Model file for the job. Use its own axes, mm. A direction names the side the tool comes from. Give positions to 0.01 mm unless a question says otherwise; leave off trailing zeros. Answer as CSV lines item,"result". Start each with the question number.
Item 1: Pull direction X, two halves, no side cores. Call faces 1 (the flat face through (86.43, -55.25, 4.78)), 2 (the flat face through (7.29, 113.98, 1.57)), 3 (the flat face through (-28.156, -69.447, 1.565)): pulls with the +X half, pulls with the -X half, needs draft (parallel to the pull), parting line crosses it, or undercut.
Item 2: Drill centre lines: L1, parallel to Y at x = 56, z = 4.5; L2, parallel to X at y = -35, z = 4; L3, parallel to X at y = 25, z = 5.5 (3 decimals). Where is each one in solid material? Low to high. Write a range as from..to.
Item 3: Tool access for faces 4 (the flat face through (-28.156, -69.447, 4.785)), 5 (the flat face through (86.43, -55.25, 1.57)), 6 (the flat face through (65.881, -68.712, 1.565)), 7 (the flat face through (-77.063, 35.143, 1.565)): list every direction of +Z, -Z, +X, -X, +Y, -Y with a clear straight run to the whole face (end or side of a thin tool).
Item 4: Pin check, flat tips, straight feed: pin 1 (1.5 mm diameter, centred on y = 87, z = 1.5, fed in from +X); pin 2 (2 mm diameter, centred on x = -66, y = 58.5, fed in from -Z); pin 3 (3 mm diameter, centred on x = 50.5, z = 3, fed in from +Y). Stop position of each tip, or through.
from build123d import *

# Parameters (mm, degrees)
F1_DEPTH = 6.35
F2_SIZE  = 3.17499


# Not quite as in the source:
# - a fillet or chamfer is up to 0.001 mm smaller than in the source, because OpenCascade refuses the exact size
# - a feature names something its author has since deleted; it is built from what else it names


with BuildPart() as f1:
    # F0 (on Top) → F1 (new body)
    with BuildSketch(Plane.XY):
        with BuildLine():
            Line((19.3683549781, 156.3463236885), (-8.1032558219, 71.7973993899))
            Line((-8.1032558219, 71.7973993899), (8.3683549781, 71.7973993899))
            ThreePointArc((8.3683549781, 71.7973993899), (11.590180385, 79.5755739829), (19.3683549781, 82.7973993899))
            Line((19.3683549781, 82.7973993899), (19.3683549781, 156.3463236885))
        make_face()
        with BuildLine():
            Line((19.3683549781, 60.7973993899), (19.3683549781, 59.7189816329))
            Line((19.3683549781, 59.7189816329), (38.0644816066, 59.7189816329))
            ThreePointArc((38.0644816066, 59.7189816329), (40.489965778, 67.183854337), (46.839965778, 71.7973993899))
            Line((46.839965778, 71.7973993899), (30.3683549781, 71.7973993899))
            ThreePointArc((30.3683549781, 71.7973993899), (27.1465295711, 64.0192247968), (19.3683549781, 60.7973993899))
        make_face()
        with BuildLine():
            Line((19.3683549781, 59.7189816329), (0.6722283496, 59.7189816329))
            ThreePointArc((0.6722283496, 59.7189816329), (-0.7119887932, 53.9533022862), (-4.5628989463, 49.4444658044))
            Line((-4.5628989463, 49.4444658044), (12.9027172029, 25.4051075068))
            ThreePointArc((12.9027172029, 25.4051075068), (15.96916804, 26.9675422479), (19.3683549781, 27.5059205686))
            Line((19.3683549781, 27.5059205686), (19.3683549781, 59.7189816329))
        make_face()
        with BuildLine():
            ThreePointArc((-4.5628989463, 49.4444658044), (-17.7934509971, 48.4031987757), (-24.7277716504, 59.7189816329))
            Line((-24.7277716504, 59.7189816329), (-29.8177793123, 44.0535488478))
            ThreePointArc((-29.8177793123, 44.0535488478), (-24.3177793123, 40.0575649437), (-22.2169662504, 33.5919271685))
            ThreePointArc((-22.2169662504, 33.5919271685), (-22.3523945039, 31.8711480531), (-22.7553445712, 30.1927402304))
            Line((-22.7553445712, 30.1927402304), (8.9067332988, 19.9051075068))
            ThreePointArc((8.9067332988, 19.9051075068), (10.46916804, 22.9715583438), (12.9027172029, 25.4051075068))
            Line((12.9027172029, 25.4051075068), (-4.5628989463, 49.4444658044))
        make_face()
        with BuildLine():
            Line((-36.6161531886, 23.1303054893), (-41.7061608505, 7.4648727041))
            ThreePointArc((-41.7061608505, 7.4648727041), (-29.4449273159, 12.5436419256), (-19.353227265, 3.9245158286))
            Line((-19.353227265, 3.9245158286), (8.9067332988, 13.1067336305))
            ThreePointArc((8.9067332988, 13.1067336305), (8.3683549781, 16.5059205686), (8.9067332988, 19.9051075068))
            Line((8.9067332988, 19.9051075068), (-22.7553445712, 30.1927402304))
            ThreePointArc((-22.7553445712, 30.1927402304), (-28.2230707533, 23.7908554024), (-36.6161531886, 23.1303054893))
        make_face()
        with BuildLine():
            ThreePointArc((-18.7316450219, 0), (-23.9667723178, -10.2745158286), (-35.3561608505, -12.0784177569))
            Line((-35.3561608505, -12.0784177569), (-22.0303477886, -21.7601876667))
            ThreePointArc((-22.0303477886, -21.7601876667), (-14.8519399659, -17.3612536953), (-6.6655230753, -19.3266385037))
            Line((-6.6655230753, -19.3266385037), (12.9027172029, 7.6067336305))
            ThreePointArc((12.9027172029, 7.6067336305), (10.46916804, 10.0402827934), (8.9067332988, 13.1067336305))
            Line((8.9067332988, 13.1067336305), (-19.353227265, 3.9245158286))
            ThreePointArc((-19.353227265, 3.9245158286), (-18.8880030964, 1.986717706), (-18.7316450219, 0))
        make_face()
        with BuildLine():
            ThreePointArc((19.3683549781, 5.5059205686), (15.96916804, 6.0442988894), (12.9027172029, 7.6067336305))
            Line((12.9027172029, 7.6067336305), (-6.6655230753, -19.3266385037))
            ThreePointArc((-6.6655230753, -19.3266385037), (-3.3300890844, -23.2319299447), (-2.1311608505, -28.2258254419))
            ThreePointArc((-2.1311608505, -28.2258254419), (-2.6695391712, -31.62501238), (-4.2319739124, -34.6914632171))
            Line((-4.2319739124, -34.6914632171), (9.0938391495, -44.3732331268))
            ThreePointArc((9.0938391495, -44.3732331268), (8.0525721209, -31.142681076), (19.3683549781, -24.2083604227))
            Line((19.3683549781, -24.2083604227), (19.3683549781, 5.5059205686))
        make_face()
        with BuildLine():
            Line((45.4022330314, -19.3266385037), (25.8339927533, 7.6067336305))
            ThreePointArc((25.8339927533, 7.6067336305), (22.7675419162, 6.0442988894), (19.3683549781, 5.5059205686))
            Line((19.3683549781, 5.5059205686), (19.3683549781, -24.2083604227))
            ThreePointArc((19.3683549781, -24.2083604227), (28.3486110991, -27.9281043016), (32.0683549781, -36.9083604227))
            ThreePointArc((32.0683549781, -36.9083604227), (31.446772735, -40.8328762512), (29.6428708066, -44.3732331268))
            Line((29.6428708066, -44.3732331268), (42.9686838685, -34.6914632171))
            ThreePointArc((42.9686838685, -34.6914632171), (41.0032990601, -26.5050463264), (45.4022330314, -19.3266385037))
        make_face()
        with BuildLine():
            ThreePointArc((29.8299766573, 13.1067336305), (28.2675419162, 10.0402827934), (25.8339927533, 7.6067336305))
            Line((25.8339927533, 7.6067336305), (45.4022330314, -19.3266385037))
            ThreePointArc((45.4022330314, -19.3266385037), (53.5886499221, -17.3612536953), (60.7670577448, -21.7601876667))
            Line((60.7670577448, -21.7601876667), (74.0928708066, -12.0784177569))
            ThreePointArc((74.0928708066, -12.0784177569), (61.188098857, -8.9802561211), (58.0899372211, 3.9245158286))
            Line((58.0899372211, 3.9245158286), (29.8299766573, 13.1067336305))
        make_face()
        with BuildLine():
            Line((61.4920545274, 30.1927402304), (29.8299766573, 19.9051075068))
            ThreePointArc((29.8299766573, 19.9051075068), (30.2329267246, 18.2266996841), (30.3683549781, 16.5059205686))
            ThreePointArc((30.3683549781, 16.5059205686), (30.2329267246, 14.7851414532), (29.8299766573, 13.1067336305))
            Line((29.8299766573, 13.1067336305), (58.0899372211, 3.9245158286))
            ThreePointArc((58.0899372211, 3.9245158286), (68.1816372721, 12.5436419256), (80.4428708066, 7.4648727041))
            Line((80.4428708066, 7.4648727041), (75.3528631447, 23.1303054893))
            ThreePointArc((75.3528631447, 23.1303054893), (66.9597807095, 23.7908554024), (61.4920545274, 30.1927402304))
        make_face()
        with BuildLine():
            Line((68.5544892685, 44.0535488478), (63.4644816066, 59.7189816329))
            ThreePointArc((63.4644816066, 59.7189816329), (56.5301609533, 48.4031987757), (43.2996089025, 49.4444658044))
            Line((43.2996089025, 49.4444658044), (25.8339927533, 25.4051075068))
            ThreePointArc((25.8339927533, 25.4051075068), (28.2675419162, 22.9715583438), (29.8299766573, 19.9051075068))
            Line((29.8299766573, 19.9051075068), (61.4920545274, 30.1927402304))
            ThreePointArc((61.4920545274, 30.1927402304), (62.1526044405, 38.5858226656), (68.5544892685, 44.0535488478))
        make_face()
        with BuildLine():
            Line((8.3683549781, 71.7973993899), (-8.1032558219, 71.7973993899))
            ThreePointArc((-8.1032558219, 71.7973993899), (-1.7532558219, 67.183854337), (0.6722283496, 59.7189816329))
            Line((0.6722283496, 59.7189816329), (19.3683549781, 59.7189816329))
            Line((19.3683549781, 59.7189816329), (19.3683549781, 60.7973993899))
            ThreePointArc((19.3683549781, 60.7973993899), (11.590180385, 64.0192247968), (8.3683549781, 71.7973993899))
        make_face()
        with BuildLine():
            Line((46.839965778, 71.7973993899), (19.3683549781, 156.3463236885))
            Line((19.3683549781, 156.3463236885), (19.3683549781, 82.7973993899))
            ThreePointArc((19.3683549781, 82.7973993899), (27.1465295711, 79.5755739829), (30.3683549781, 71.7973993899))
            Line((30.3683549781, 71.7973993899), (46.839965778, 71.7973993899))
        make_face()
        with BuildLine():
            Line((38.0644816066, 59.7189816329), (19.3683549781, 59.7189816329))
            Line((19.3683549781, 59.7189816329), (19.3683549781, 27.5059205686))
            ThreePointArc((19.3683549781, 27.5059205686), (22.7675419162, 26.9675422479), (25.8339927533, 25.4051075068))
            Line((25.8339927533, 25.4051075068), (43.2996089025, 49.4444658044))
            ThreePointArc((43.2996089025, 49.4444658044), (39.4486987494, 53.9533022862), (38.0644816066, 59.7189816329))
        make_face()
        with BuildLine():
            Line((-29.8177793123, 44.0535488478), (-24.7277716504, 59.7189816329))
            Line((-24.7277716504, 59.7189816329), (-113.6277716504, 59.7189816329))
            Line((-113.6277716504, 59.7189816329), (-43.6785879297, 36.9911141066))
            ThreePointArc((-43.6785879297, 36.9911141066), (-38.2108617476, 43.3929989346), (-29.8177793123, 44.0535488478))
        make_face()
        with BuildLine():
            Line((-43.6785879297, 36.9911141066), (-113.6277716504, 59.7189816329))
            Line((-113.6277716504, 59.7189816329), (-41.7061608505, 7.4648727041))
            Line((-41.7061608505, 7.4648727041), (-36.6161531886, 23.1303054893))
            ThreePointArc((-36.6161531886, 23.1303054893), (-43.0180380165, 28.5980316714), (-43.6785879297, 36.9911141066))
        make_face()
        with BuildLine():
            Line((-22.0303477886, -21.7601876667), (-35.3561608505, -12.0784177569))
            Line((-35.3561608505, -12.0784177569), (-62.8277716504, -96.6273420556))
            Line((-62.8277716504, -96.6273420556), (-19.5967986257, -37.12501238))
            ThreePointArc((-19.5967986257, -37.12501238), (-23.995732597, -29.9466045573), (-22.0303477886, -21.7601876667))
        make_face()
        with BuildLine():
            Line((-19.5967986257, -37.12501238), (-62.8277716504, -96.6273420556))
            Line((-62.8277716504, -96.6273420556), (9.0938391495, -44.3732331268))
            Line((9.0938391495, -44.3732331268), (-4.2319739124, -34.6914632171))
            ThreePointArc((-4.2319739124, -34.6914632171), (-11.410381735, -39.0903971884), (-19.5967986257, -37.12501238))
        make_face()
        with BuildLine():
            ThreePointArc((58.3335085819, -37.12501238), (50.1470916912, -39.0903971884), (42.9686838685, -34.6914632171))
            Line((42.9686838685, -34.6914632171), (29.6428708066, -44.3732331268))
            Line((29.6428708066, -44.3732331268), (101.5644816066, -96.6273420556))
            Line((101.5644816066, -96.6273420556), (58.3335085819, -37.12501238))
        make_face()
        with BuildLine():
            Line((74.0928708066, -12.0784177569), (60.7670577448, -21.7601876667))
            ThreePointArc((60.7670577448, -21.7601876667), (62.3294924859, -24.8266385037), (62.8678708066, -28.2258254419))
            ThreePointArc((62.8678708066, -28.2258254419), (61.6689425727, -33.219720939), (58.3335085819, -37.12501238))
            Line((58.3335085819, -37.12501238), (101.5644816066, -96.6273420556))
            Line((101.5644816066, -96.6273420556), (74.0928708066, -12.0784177569))
        make_face()
        with BuildLine():
            Line((80.4428708066, 7.4648727041), (152.3644816066, 59.7189816329))
            Line((152.3644816066, 59.7189816329), (82.4152978859, 36.9911141066))
            ThreePointArc((82.4152978859, 36.9911141066), (82.8182479532, 35.312706284), (82.9536762066, 33.5919271685))
            ThreePointArc((82.9536762066, 33.5919271685), (80.8528631447, 27.1262893933), (75.3528631447, 23.1303054893))
            Line((75.3528631447, 23.1303054893), (80.4428708066, 7.4648727041))
        make_face()
        with BuildLine():
            Line((152.3644816066, 59.7189816329), (63.4644816066, 59.7189816329))
            Line((63.4644816066, 59.7189816329), (68.5544892685, 44.0535488478))
            ThreePointArc((68.5544892685, 44.0535488478), (76.9475717037, 43.3929989346), (82.4152978859, 36.9911141066))
            Line((82.4152978859, 36.9911141066), (152.3644816066, 59.7189816329))
        make_face()
    extrude(amount=F1_DEPTH)

    # F2 (size 3.175 in the source; OpenCascade refuses exactly that, so slightly less here)
    f2_edges = [f1.edges().sort_by_distance(p)[0] for p in [
        (-77.666966, 33.591927, 6.35),
        (-69.177772, 59.718982, 6.35),
        (5.63255, 114.071862, 6.35),
        (33.10416, 114.071862, 6.35),
        (107.914482, 59.718982, 6.35),
        (116.403676, 33.591927, 6.35),
        (87.828676, -54.35288, 6.35),
        (65.603676, -70.500288, 6.35),
        (-26.866966, -70.500288, 6.35),
        (-49.091966, -54.35288, 6.35),
        (-26.866966, -70.500288, 0),
        (-49.091966, -54.35288, 0),
        (65.603676, -70.500288, 0),
        (87.828676, -54.35288, 0),
        (116.403676, 33.591927, 0),
        (107.914482, 59.718982, 0),
        (33.10416, 114.071862, 0),
        (5.63255, 114.071862, 0),
        (-69.177772, 59.718982, 0),
        (-77.666966, 33.591927, 0),
    ]]
    chamfer(f2_edges, length=F2_SIZE)


solid = f1.part
Responses:
1,face 1,"pulls with the +X half"
1,face 2,"pulls with the -X half"
1,face 3,"undercut"
2,L1,"-61.89..-38.42, -18.03..48.15"
2,L2,"-41.94..-21.8, -4.46..6.81, 31.92..43.2, 60.53..80.67"
2,L3,"-61.886..-40.086, -26.348..12.379, 26.358..65.085, 78.822..100.622"
3,face 4,"+Z, -Y"
3,face 5,"-Z, +X"
3,face 6,"-Z, -Y"
3,face 7,"-Z, -X"
4,pin 1,"x = 40.96"
4,pin 2,"z = 0.96"
4,pin 3,"y = 47.14"
